Autodesk Inventor part; units mm, degrees
ref_plane "Work Plane1" through (5, 0, 0) normal (0, -0.5, -0.866) x (1, 0, 0)
ref_plane "YZ Plane" through (0, 0, 0) normal (1, 0, 0) x (0, 1, 0)
ref_plane "XZ Plane" through (0, 0, 0) normal (0, 1, 0) x (-1, 0, 0)
sketch "Sketch1" plane through (0, 0, 0) normal (0, 0, 1) x (1, 0, 0)
  line L0 (0.4041, 0) -> (7.5, 0)
  line L1 (10, 0.866) -> (10, 1.5)
  line L2 (10, 1.5) -> (0, 1.5)
  line L3 (10, 0.866) -> (8, 0.866)
  line L4 (8, 0.866) -> (7.5, 0)
  line L5 (0, 0.7) -> (0.4041, 0)
  line L6 (0, -0.3) -> (0, 1.8)
  line L7 (0, 0.7) -> (0, 1.5)
  point P0 (0, 0)
  dimension "d0" = 2
  dimension "d1" = 60
  dimension "d2" = 3
  dimension "d3" = 1.7321
  dimension "d4" = 10
  dimension "d5" = 60
  dimension "d7" = 1.4
revolve "Body" add sketch "Sketch1" angle 360 about axis through (0.4041, 0, 0) along (1, 0, 0)
sketch "Sketch2" plane through (10, 0, 0) normal (1, 0, 0) x (0, 0, -1)
  circle A0 centre (0, 0) radius 0.866
  circle A1 centre (0, 0) radius 1.5
  line L0 (0.866, 0) -> (0.433, -0.75)
  line L1 (0.433, -0.75) -> (-0.433, -0.75)
  line L2 (-0.433, -0.75) -> (-0.866, 0)
  line L3 (-0.866, 0) -> (-0.433, 0.75)
  line L4 (-0.433, 0.75) -> (0.433, 0.75)
  line L5 (0.433, 0.75) -> (0.866, 0)
extrude "Slot" add sketch "Sketch2" against normal blind 2 contours L5 A0 | A0 L0 | L4 A0 | A0 L1 | L3 A0 | A0 L2
chamfer "Chamfer1" distance 0.8 angle 45 1 edges at (0, -1.5, 0) measured on face at (0, 1.2188, -0.1197)
thread "Thread"
chamfer "Chamfer2" distance 0.3067 angle 45 1 edges at (10, -1.5, 0) measured on face at (3.8663, 1.4806, -0.2406)
ref_plane "Work Plane1" through (5, 0, 0) normal (0, -0.5, -0.866) x (1, 0, 0)
equation "\"d0\" = INTI"
equation "\"d2\" = NND"
equation "\"d3\" = 1.1547 * SW"
equation "\"d4\" = NLG"
equation "\"d5\" = 0.5 * ANG"
equation "\"d7\" = SPD"
equation "\"d8\" = INTI"
equation "\"d10\" = -0.5 * SPD + 0.5 * NND"
equation "\"d11\" = FAWI"
equation "\"d33\" = -0.5 * SPD + 0.5 * NND"
equation "\"d14\" = NLG"
equation "\"d12\" = -0.5 * GD1 + 0.5 * NND"
equation "\"d13\" = FAWI"
equation "\"d34\" = -0.5 * GD1 + 0.5 * NND"
equation "\"NND\" = 3"
equation "\"NLG\" = 10"
equation "\"INTI\" = 2"
equation "\"FAWI\" = 45deg"
equation "\"SW\" = 1.5"
equation "\"GD1\" = THREADDIA - 1.2269 * PTC"
equation "\"ANG\" = 120deg"
equation "\"FAWI1\" = 45deg"
equation "\"SPD\" = 1.4"
equation "\"GUL\" = 0.61345 * PTC"
equation "\"TOA\" = 30deg"
equation "\"THREADDIA\" = 3"
equation "\"PTC\" = 0.5"
equation "\"GAL\" = 0.61345 * PTC"
equation "\"E0\" = 1.155 * SW"
properties part number "DIN 916 - M3  x  10" material "Steel, Mild"
Geometry check sheet. Reference: the model listing, model coordinates, mm. A direction names the side the tool comes from. Give positions to 0.01 mm unless a question says otherwise; leave off trailing zeros. Order: outer loops, then holes, each group sorted by start corner. A loop starts at its lowest first (then second) coordinate and runs counter-clockwise, first axis right, second up. Notation, with made-up numbers: (30.25, 26) - (34.25, 26) arc R26 ccw to (34.25, 51) - close; hole circle Ø11 at (-3, -10). An arc over 180 degrees is marked (long way). Answer as a JSON object with one key per item and string values.
(1) Material ranges on line 1 (Z direction, x = 3.75, y = 1.3); line 2 (Z direction, x = 9.5, y = -0.4); line 3 (Z direction, x = 8.5, y = 0.05), recorded low to high.
Report:
{"line 1": "-0.75 to 0.75", "line 2": "-1.45 to -0.64, 0.64 to 1.45", "line 3": "-1.5 to -0.84, 0.84 to 1.5"}
(2) Cross-section at A-A (x = 4.5). Record the cut outline in (y, z), then the cut area to 3 significant figures.
Report:
{"outline": "circle Ø3 at (0, 0)", "area": "7.07 mm^2"}
(3) Depth check by flat-ended pin: pin 1 Ø1.5 at (x, y) = (8.5, -1) entering from +Z; pin 2 Ø0.5 at (y, z) = (0.5, 1) entering from -X. Enter the tip coordinate at first touch or a pass-through.
Report:
{"pin 1": "z = 1.48", "pin 2": "x = 0.17"}
(4) Tool access check on faces 4 (the flat face through (9, 0.75, 0)), 5 (the conical face through (0.334, -0.026, 0.119)). Record the directions out of +Z, -Z, +X, -X, +Y, -Y that give a thin tool (end or side, any length) a straight path to the whole face; none if there is none.
Report:
{"face 4": "+X", "face 5": "-X"}
(5) Draft check along Z on faces 1 (the cylindrical face through (5.18, -1.5, -0.07)), 2 (the flat face through (9, -0.75, 0)), 3 (the flat face through (10, 1, 0)). Enter one of: released by +Z, released by -Z, zero draft, split by the parting line, or undercut.
Report:
{"face 1": "split by the parting line", "face 2": "undercut", "face 3": "zero draft"}
